For this review, take the finished solid that the model builds, in its own axes (mm). A direction names the side the tool comes from. Give positions to 0.01 mm unless a question says otherwise; leave off trailing zeros. Order: outer loops, then holes, each group sorted by start corner. A loop starts at its lowest first (then second) coordinate and runs counter-clockwise, first axis right, second up. Notation, with made-up numbers: (11.25, 81) -> (64.25, 81) arc R31 cw to (64.25, 113) -> close; hole circle Ø8 at (-1.75, -12). An arc over 180 degrees is marked (long way). Return JSON: item names as keys, results as strings. Group by question number.
1) The part is to be moulded in two halves that separate along Y. For faces 4 (the face through (10.808, 4.873, -2.471)), 5 (the face through (9, 6, 0)), 6 (the face through (13, 4, -1.584)), 7 (the face through (5, 4.8, 4)), say which applies: released by +Y, released by -Y, zero draft, split by the parting line, or undercut.
2) Add section A-A (y = 1). Give the boundary of the cut face in (x, z).
3) For faces 1 (the face through (9.076, 1, 0)), 2 (the face through (6.073, 5.894, -2.471)), 3 (the face through (0.682, 2, 2)), list the 3-axis set-ups (+Z, -Z, +X, -X, +Y, -Y) from which the entire face can be reached by the end or side of a thin tool; tool diameter is ignored.
4) Add section B-B (y = 3.95). Give the boundary of the cut face in (x, z), then the cut area to 3 significant figures.
5) Add section D-D (y = 2.75). Give the boundary of the cut face in (x, z), then the cut area to 3 significant figures.
6) To check wall thickness, follow line 1 along X through (y, z) = (0.5, 0.5); line 2 along X through (y, z) = (3.15, 4); line 3 along X through (y, z) = (1.05, 4). State the ranges of each line that lie inside material, in increasing order.
7) Insertion check: P1, Ø2, axis at x = 9, z = 2.5, coming from the -Y side; P2, Ø2.5, axis at x = 13, z = 4, coming from the -Y side; P3, Ø4, axis at x = 9, z = 3, coming from the -Y side. Each pin has a flat end and moves straight along its axis. Give the tip position at first contact, or say it passes through.
from build123d import *

# Parameters (mm, degrees)
MAINBASESKETCH_W             = 15.8
MAINBASESKETCH_H             = 3.2
MAINBASEEXTRUDE_DEPTH        = 7.9
STUDSSKETCH_R                = 2.3
STUDSEXTRUDE_DEPTH           = 1.6
STUDSPATTERN_COUNT           = 2
STUDSPATTERN_PITCH           = 8
STUDSPATTERN_COUNT_DIR2      = 2
STUDSPATTERN_PITCH_DIR2      = 8
MAINBASESHELL_T              = -1.2
LCUTBLUE_DEPTH               = 19.555463972
LCUTBLUE_DEPTH_BACK          = 19.555463972
CUTADDEDTOLCUT_DEPTH         = 2
MADESLIMCUTSKETCH_W          = 7.9
MADESLIMCUTSKETCH_H          = 7.9
MADESLIMCUT_DEPTH            = 19.897228453
MADESLIMFILLEXT_REACH        = 20.897
SKETCH33_W                   = 5.500952983
SKETCH33_H                   = 1.199047018
SLIMHOLEEXT_START            = -0.2
SLIMHOLESKETCH_R             = 1.75
SLIMHOLESKETCH_R_2           = 0.75
SLIMHOLEEXT_DEPTH            = 2
SHORTLEXTENSIONSKETCH_W      = 1.583745828
SHORTLEXTENSIONSKETCH_H      = 7.9
SHORTLEXTENDEDCUTSKETCH_W    = 13.4
SHORTLEXTENDEDCUTSKETCH_H    = 1.582792846
SHORTLEXTENDEDCUT_DEPTH      = 2
SHORTLUNDERSTUMPS_START      = -0.2
SHORTLUNDERSTUMPSKETCH_W     = 0.996828098
SHORTLUNDERSTUMPSKETCH_H     = 1.5
SHORTLUNDERSTUMPS_DEPTH      = 2.15
SHORTLUPPERCIRCLES_START     = -0.2
SHORTLUPPERCIRCLESSKETCH_R   = 2.45
SHORTLUPPERCIRCLESSKETCH_R_2 = 2
SHORTLUPPERCIRCLES_DEPTH     = 2


with BuildPart() as part:
    # MainBaseSketch → MainBaseExtrude (new, symmetric)
    with BuildSketch(Plane.XY):
        with Locations((8.581967213, 1.6)):
            Rectangle(MAINBASESKETCH_W, MAINBASESKETCH_H)
    extrude(amount=MAINBASEEXTRUDE_DEPTH, both=True)

    # StudsSketch → StudsExtrude (add)
    with BuildSketch(Plane(origin=(0, 3.2, 0), x_dir=(1, 0, 0), z_dir=(0, 1, 0))):
        with Locations(Location((4.581967213, 4, 0), (0, 0, 90))):
            Circle(STUDSSKETCH_R)
    studsextrude = extrude(amount=STUDSEXTRUDE_DEPTH)

    # StudsPattern: StudsExtrude 2 × 2
    with Locations(*[(j * STUDSPATTERN_PITCH_DIR2, 0, i * STUDSPATTERN_PITCH) for i in range(STUDSPATTERN_COUNT) for j in range(STUDSPATTERN_COUNT_DIR2) if (i, j) != (0, 0)]):
        add(studsextrude)

    # MainBaseShell
    mainbaseshell_openings = [part.faces().sort_by_distance(p)[0] for p in [
        (8.581967213, 0, 0),
    ]]
    offset(amount=MAINBASESHELL_T, openings=mainbaseshell_openings, kind=Kind.INTERSECTION)

    # LCUTBlueSketch → LCutBlue (cut, two sides: drawn at the far end of the back side and taken through both)
    with BuildSketch(Plane(origin=(0, 3.2, 0), x_dir=(1, 0, 0), z_dir=(0, 1, 0)).offset(-LCUTBLUE_DEPTH_BACK)):
        Polygon((8.581967213, 53.229874044), (8.581967213, 7.9), (8.581967213, 0), (16.481967213, 0), (61.811841258, 0), (125.917963912, 64.106122654), (72.688089868, 117.335996699), align=None)
    extrude(amount=LCUTBLUE_DEPTH + LCUTBLUE_DEPTH_BACK, mode=Mode.SUBTRACT)

    # CutAddedtoLSketch → CutAddedToLCut (add)
    with BuildSketch(Plane.XZ):
        Polygon((7.382920196, -6.7), (8.581967213, -6.7), (8.581967213, 0), (15.281967213, 0), (15.281967213, 1.199047018), (7.382920196, 1.199047018), (7.382920196, 0), align=None)
    extrude(amount=-CUTADDEDTOLCUT_DEPTH)

    # MadeSlimCutSketch → MadeSlimCut (cut, through all)
    with BuildSketch(Plane.XZ):
        with Locations((4.631967213, -3.95)):
            Rectangle(MADESLIMCUTSKETCH_W, MADESLIMCUTSKETCH_H)
    extrude(amount=-MADESLIMCUT_DEPTH, mode=Mode.SUBTRACT)

    # Sketch33 → MadeSlimFillExt (add, up to next)
    with BuildSketch(Plane.XZ, mode=Mode.PRIVATE) as madeslimfillext_sk1:
        with Locations((4.632443704, 0.599523509)):
            Rectangle(SKETCH33_W, SKETCH33_H)
    madeslimfillext_tool1 = extrude(madeslimfillext_sk1.sketch, amount=-MADESLIMFILLEXT_REACH, mode=Mode.PRIVATE) - part.part
    add(madeslimfillext_tool1.solids().sort_by_distance((4.632444, 0, 0.599524))[0])

    # SlimHoleSketch → SlimHoleExt (add)
    with BuildSketch(Plane.XZ.offset(-2).offset(SLIMHOLEEXT_START)):
        with Locations(Location((8.581967213, 4, 0), (0, 0, 270))):
            Circle(SLIMHOLESKETCH_R)
        with Locations(Location((8.581967213, 4, 0), (0, 0, 270))):
            Circle(SLIMHOLESKETCH_R_2, mode=Mode.SUBTRACT)
    extrude(amount=SLIMHOLEEXT_DEPTH)

    # ShortLExtension: sweep along a curve in space
    with BuildLine() as shortlextension_path:
        Line((0.681967213, 3.2, 0), (16.481967213, 3.2, 0))
    # ShortLExtensionSketch → ShortLExtension (sweep)
    with BuildSketch(Plane(origin=(16.481967213, 0, 0), x_dir=(0, 0, -1), z_dir=(1, 0, 0))):
        with Locations((0.791872914, 3.95)):
            Rectangle(SHORTLEXTENSIONSKETCH_W, SHORTLEXTENSIONSKETCH_H)
    sweep(path=shortlextension_path.line)

    # ShortLExtendedCutSketch → ShortLExtendedCut (cut)
    with BuildSketch(Plane.XZ):
        with Locations((8.581967213, 0.407650595)):
            Rectangle(SHORTLEXTENDEDCUTSKETCH_W, SHORTLEXTENDEDCUTSKETCH_H)
    extrude(amount=-SHORTLEXTENDEDCUT_DEPTH, mode=Mode.SUBTRACT)

    # ShortLUnderStumpSketch → ShortLUnderStumps (add)
    with BuildSketch(Plane.XZ.offset(-2).offset(SHORTLUNDERSTUMPS_START)):
        with Locations((4.581764801, 0.366254172)):
            Rectangle(SHORTLUNDERSTUMPSKETCH_W, SHORTLUNDERSTUMPSKETCH_H)
        with Locations((8.57767054, 0.366254172)):
            Rectangle(SHORTLUNDERSTUMPSKETCH_W, SHORTLUNDERSTUMPSKETCH_H)
        with Locations((12.582169625, 0.366254172)):
            Rectangle(SHORTLUNDERSTUMPSKETCH_W, SHORTLUNDERSTUMPSKETCH_H)
    extrude(amount=SHORTLUNDERSTUMPS_DEPTH)

    # ShortLUpperCirclesSketch → ShortLUpperCircles (add)
    # profile 1 of 2: a face of its own
    with BuildSketch(Plane(origin=(0, 0, -1.583745828), x_dir=(-1, 0, 0), z_dir=(0, 0, -1)).offset(SHORTLUPPERCIRCLES_START)):
        with Locations(Location((-12.581967213, 3.95, 0), (0, 0, 90))):
            Circle(SHORTLUPPERCIRCLESSKETCH_R)
        with Locations(Location((-12.581967213, 3.95, 0), (0, 0, 90))):
            Circle(SHORTLUPPERCIRCLESSKETCH_R_2, mode=Mode.SUBTRACT)
    # profile 2 of 2: a face of its own
    with BuildSketch(Plane(origin=(0, 0, -1.583745828), x_dir=(-1, 0, 0), z_dir=(0, 0, -1)).offset(SHORTLUPPERCIRCLES_START)):
        with Locations(Location((-4.581967213, 3.95, 0), (0, 0, 270))):
            Circle(SHORTLUPPERCIRCLESSKETCH_R)
        with Locations(Location((-4.581967213, 3.95, 0), (0, 0, 270))):
            Circle(SHORTLUPPERCIRCLESSKETCH_R_2, mode=Mode.SUBTRACT)
    extrude(amount=SHORTLUPPERCIRCLES_DEPTH)


solid = part.part
Evaluation:
{
 "1": {"face 4": "undercut", "face 5": "zero draft", "face 6": "undercut", "face 7": "released by +Y"},
 "2": {"outline": "(0.68, -1.58) -> (16.48, -1.58) -> (16.48, 7.9) -> (0.68, 7.9) -> close; circle Ø3.5 at (8.58, 4); hole (1.88, -0.38) -> (4.08, -0.38) -> (4.08, 1.12) -> (5.08, 1.12) -> (5.08, -0.38) -> (8.08, -0.38) -> (8.08, 1.12) -> (9.08, 1.12) -> (9.08, -0.38) -> (12.08, -0.38) -> (12.08, 1.12) -> (13.08, 1.12) -> (13.08, -0.38) -> (15.28, -0.38) -> (15.28, 6.7) -> (1.88, 6.7) -> close; hole circle Ø1.5 at (8.58, 4)"},
 "3": {"face 1": "-Y", "face 2": "-Z", "face 3": "+Z, -Z, -X, +Y, -Y"},
 "4": {"outline": "(0.68, -1.58) -> (2.13, -1.58) -> (2.13, -3.38) -> (2.58, -3.38) -> (2.58, -1.58) -> (6.58, -1.58) -> (6.58, -3.38) -> (7.03, -3.38) -> (7.03, -1.58) -> (10.13, -1.58) -> (10.13, -3.38) -> (10.58, -3.38) -> (10.58, -1.58) -> (14.58, -1.58) -> (14.58, -3.38) -> (15.03, -3.38) -> (15.03, -1.58) -> (16.48, -1.58) -> (16.48, 0) -> (0.68, 0) -> close; circle Ø4.6 at (4.58, 4); circle Ø4.6 at (12.58, 4)", "area": "61.5 mm^2"},
 "5": {"outline": "(0.68, -1.58) -> (2.45, -1.58) -> (2.45, -3.38) -> (2.98, -3.38) -> (2.98, -1.58) -> (6.18, -1.58) -> (6.18, -3.38) -> (6.72, -3.38) -> (6.72, -1.58) -> (10.45, -1.58) -> (10.45, -3.38) -> (10.98, -3.38) -> (10.98, -1.58) -> (14.18, -1.58) -> (14.18, -3.38) -> (14.72, -3.38) -> (14.72, -1.58) -> (16.48, -1.58) -> (16.48, 7.9) -> (0.68, 7.9) -> close; hole circle Ø2.2 at (4.58, 4); hole circle Ø2.2 at (12.58, 4)", "area": "146 mm^2"},
 "6": {"line 1": "0.68 to 1.88, 4.08 to 5.08, 8.08 to 9.08, 12.08 to 13.08, 15.28 to 16.48", "line 2": "0.68 to 3.48, 5.68 to 11.48, 13.68 to 16.48", "line 3": "0.68 to 1.88, 6.83 to 7.83, 9.33 to 10.33, 15.28 to 16.48"},
 "7": {"P1": "y = 0.2", "P2": "y = 2", "P3": "y = 0.05"}
}
